For this review, take the finished solid that the model builds, in its own axes (mm). A direction names the side the tool comes from. Coordinates: 2 decimals unless noted, no trailing zeros. Loops run counter-clockwise (first coordinate to the right, second up) from the corner with the lowest first, then second, coordinate; pieces in that order, holes last. Notation, with made-up numbers: (29, 2.25) - (60, 2.25) arc R33 cw to (60, 32.25) - close; hole circle Ø3 at (33.5, 7.5). An arc over 180 degrees is marked (long way). Use one line per item in the form item = value. Start each with the question number.
1. Add section C-C on z = 27.5. Give the boundary of the cut face in (x, y) (3 decimals).
2. Add section B-B on z = 11. Give the boundary of the cut face in (x, y) (3 decimals).
3. Add section D-D on y = -20.5. Give the boundary of the cut face in (x, z).
4. Draft analysis for pull direction Y (two halves, no side actions). For faces 4 (the face through (0.18, 17.52, -20.33)), 5 (the face through (-12.7, -2, 0)), 6 (the face through (0, 33.655, 0)), 7 (the face through (0, 44.45, 0)), state which applies: +Y half, -Y half, draft (parallel to the pull), parting line (faces both ways), or undercut.
5. To check wall thickness, follow probe 1 along X at (y, z) = (-40.5, 0) (3 decimals); probe 2 along Y at (x, z) = (11.5, 4) (3 decimals); probe 3 along Y at (x, z) = (-20, -14.5). State the ranges of each line that lie inside material, in increasing order.
6. Add section A-A on x = -4.5. Give the boundary of the cut face in (y, z) (3 decimals).
7. For pin 1 Ø10.5 at (x, z) = (23, -11.5) entering from +Y; pin 2 Ø5 at (y, z) = (-7.5, -16.5) entering from -X; pin 3 Ø2 at (x, y) = (7.5, 33) entering from +Z; pin 4 Ø10 at (x, z) = (-22.225, 0) entering from -Y, all flat-tipped, find the tip position at first contact; note any pin that passes through.
8. Machinability: for faces 1 (the face through (0.18, 18.04, 20.33)), 2 (the face through (12.7, -2, 0)), 3 (the face through (-26, -38.1, 0)), which of the approach directions +Z, -Z, +X, -X, +Y, -Y give a long, thin tool a straight path to every point of the face, cutting with its end or side? Answer none if there is none.
```python
from build123d import *

# Parameters (mm, degrees)
SKETCH1_W           = 63.5
SKETCH1_H           = 88.9
BOSS_EXTRUDE1_DEPTH = 12.7
SKETCH2_W           = 63.5
SKETCH2_H           = 6.35
BOSS_EXTRUDE2_DEPTH = 28.575
FILLET1_R           = 6.35
SKETCH3_R           = 3.175
CUT_EXTRUDE1_DEPTH  = 93.946735419
FILLET2_R           = 19.05


with BuildPart() as part:
    # Sketch1 → Boss-Extrude1 (new, symmetric)
    with BuildSketch(Plane(origin=(0, 0, 0), x_dir=(0, 0, -1), z_dir=(1, 0, 0))):
        Rectangle(SKETCH1_W, SKETCH1_H)
        with BuildLine():
            Line((-12.7, 1.905), (12.7, 1.905))
            ThreePointArc((12.7, 1.905), (20.329919454, 17.78), (12.7, 33.655))
            Line((12.7, 33.655), (-12.7, 33.655))
            ThreePointArc((-12.7, 33.655), (-20.329919454, 17.78), (-12.7, 1.905))
        make_face(mode=Mode.SUBTRACT)
    extrude(amount=BOSS_EXTRUDE1_DEPTH, both=True)

    # Sketch2 → Boss-Extrude2 (add, symmetric)
    with BuildSketch(Plane(origin=(0, 0, 0), x_dir=(0, 0, -1), z_dir=(1, 0, 0))):
        with Locations((0, -41.275)):
            Rectangle(SKETCH2_W, SKETCH2_H)
    extrude(amount=BOSS_EXTRUDE2_DEPTH, both=True)

    # Fillet1
    fillet1_edges = [part.edges().sort_by_distance(p)[0] for p in [
        (12.7, -38.1, 0),
        (-12.7, -38.1, 0),
    ]]
    fillet(fillet1_edges, radius=FILLET1_R)

    # Sketch3 → Cut-Extrude1 (cut, through all)
    with BuildSketch(Plane(origin=(0, -38.1, 0), x_dir=(1, 0, 0), z_dir=(0, 1, 0))):
        with Locations(Location((22.225, 0, 0), (0, 0, 270))):
            Circle(SKETCH3_R)
    cut_extrude1 = extrude(amount=-CUT_EXTRUDE1_DEPTH, mode=Mode.SUBTRACT)

    # Mirror1: Cut-Extrude1 across plane
    add(cut_extrude1.mirror(Plane(origin=(0, 0, 0), x_dir=(0, 0, 1), z_dir=(1, 0, 0))), mode=Mode.SUBTRACT)

    # Fillet2
    fillet2_edges = [part.edges().sort_by_distance(p)[0] for p in [
        (0, 44.45, 31.75),
        (0, 44.45, -31.75),
    ]]
    fillet(fillet2_edges, radius=FILLET2_R)


solid = part.part
```
Conclusion:
q1.outline = (-28.575, -44.45) - (28.575, -44.45) - (28.575, -38.1) - (19.05, -38.1) arc R6.35 cw to (12.7, -31.75) - (12.7, 37.394) - (-12.7, 37.394) - (-12.7, -31.75) arc R6.35 cw to (-19.05, -38.1) - (-28.575, -38.1) - close
q2.outline = (-28.575, -44.45) - (28.575, -44.45) - (28.575, -38.1) - (19.05, -38.1) arc R6.35 cw to (12.7, -31.75) - (12.7, 1.905) - (-12.7, 1.905) - (-12.7, -31.75) arc R6.35 cw to (-19.05, -38.1) - (-28.575, -38.1) - close; (-12.7, 33.655) - (12.7, 33.655) - (12.7, 44.45) - (-12.7, 44.45) - close
q3.outline = (-12.7, -31.75) - (12.7, -31.75) - (12.7, 31.75) - (-12.7, 31.75) - close
q4.face_4 = undercut
q4.face_5 = draft
q4.face_6 = undercut
q4.face_7 = +Y half
q5.probe_1 = -28.575 to -25.4, -19.05 to 19.05, 25.4 to 28.575
q5.probe_2 = -44.45 to 1.905, 33.655 to 44.45
q5.probe_3 = -44.45 to -38.1
q6.outline = (-44.45, -31.75) - (25.4, -31.75) arc R19.05 ccw to (44.45, -12.7) - (44.45, 12.7) arc R19.05 ccw to (25.4, 31.75) - (-44.45, 31.75) - close; hole (1.905, -12.7) arc R20.33 ccw to (33.655, -12.7) - (33.655, 12.7) arc R20.33 ccw to (1.905, 12.7) - close
q7.pin_1 = -37.97
q7.pin_2 = -12.7
q7.pin_3 = 30.57
q7.pin_4 = -44.45
q8.face_1 = +X, -X
q8.face_2 = +Z, -Z, +X, +Y
q8.face_3 = +Z, -Z, -X, +Y
